Build history of the part. All positions in model axes, mm. Face numbers are marked on the shaded views. A direction names the side the tool comes from. Give positions to 0.01 mm unless a question says otherwise; leave off trailing zeros. Order: outer loops, then holes, each group sorted by start corner. A loop starts at its lowest first (then second) coordinate and runs counter-clockwise, first axis right, second up. Notation, with made-up numbers: (87.5, 14.25) - (129.5, 14.25) arc R21 cw to (129.5, 41.25) - close; hole circle Ø6 at (-13, 36.25). An arc over 180 degrees is marked (long way). Write each question's results on one line, items separated by ' | '. Start each with the question number.
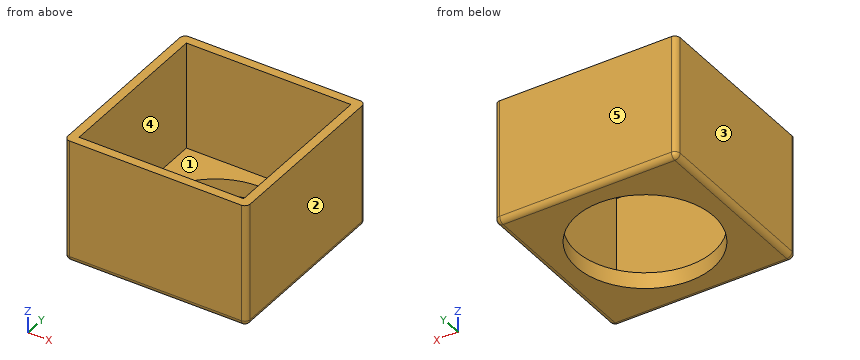
from build123d import *

# Parameters (mm, degrees)
F0_W     = 34
F0_H     = 34
F0_W_2   = 30.67
F0_H_2   = 30.67
F0_R     = 14.3
F0_R_2   = 12.8
F1_DEPTH = 3
F2_DEPTH = 20
F3_R     = 1


with BuildPart() as f1:
    # F0 (on Top) → F1 (new body)
    with BuildSketch(Plane.XY):
        Rectangle(F0_W, F0_H)
        Rectangle(F0_W_2, F0_H_2, mode=Mode.SUBTRACT)
        Rectangle(F0_W_2, F0_H_2)
        Circle(F0_R, mode=Mode.SUBTRACT)
        Circle(F0_R)
        Circle(F0_R_2, mode=Mode.SUBTRACT)
    extrude(amount=-F1_DEPTH)

    # F0 (on Top) → F2 (join)
    with BuildSketch(Plane.XY):
        Rectangle(F0_W, F0_H)
        Rectangle(F0_W_2, F0_H_2, mode=Mode.SUBTRACT)
    extrude(amount=F2_DEPTH)

    # F3
    f3_edges = [f1.edges().sort_by_distance(p)[0] for p in [
        (17, 0, -3),
        (0, 17, -3),
        (-17, 0, -3),
        (0, -17, -3),
        (17, -17, 8.5),
        (17, 17, 8.5),
        (-17, 17, 8.5),
        (-17, -17, 8.5),
    ]]
    fillet(f3_edges, radius=F3_R)


solid = f1.part
Item 1: Two-plate mould, pull along X, no slides. Class the marked faces 1, 2 and 3: +X half, -X half, draft (parallel to the pull), parting line (faces both ways), or undercut.
Item 2: Probe line 1 along X through (y, z) = (6, 5) (3 decimals); line 2 along Y through (x, z) = (0, -1.55). List the from-to ranges inside material, lowest first. Write a range as from..to.
Item 3: Cut at D-D, the plane x = 14. List the corners of the cut face in (y, z) (3 decimals), then the cut area to 3 significant figures.
Item 4: Which spindle directions (+Z, -Z, +X, -X, +Y, -Y) get a long thin tool onto all of the face, cutting with end or side? Do the marked faces 4 and 5. Say none if no direction does.
Item 5: Cut at A-A, the plane x = 0. List the corners of the cut face in (y, z) (3 decimals), then the cut area to 3 significant figures.
Item 6: Flat gauge pin, fed straight in: pin 1 Ø3 at (x, y) = (12, -10) entering from +Z. Where does the tip first touch, or does it go through?
Item 7: Cut at C-C, the plane z = 6.5. List the corners of the cut face in (x, y) (3 decimals), then the cut area to 3 significant figures.
Values found:
1) face 1: undercut | face 2: +X half | face 3: -X half
2) line 1: x = -17..-15.335, 15.335..17 | line 2: y = -17..-12.8, 12.8..17
3) outline: (-17, -2) arc R1 ccw to (-16, -3) - (16, -3) arc R1 ccw to (17, -2) - (17, 20) - (15.335, 20) - (15.335, 0) - (-15.335, 0) - (-15.335, 20) - (-17, 20) - close | area: 168 mm2
4) face 4: +Z | face 5: +Z, -Z, +X, -X, +Y
5) outline: (-17, -2) arc R1 ccw to (-16, -3) - (-12.8, -3) - (-12.8, 0) - (-15.335, 0) - (-15.335, 20) - (-17, 20) - close; (12.8, -3) - (16, -3) arc R1 ccw to (17, -2) - (17, 20) - (15.335, 20) - (15.335, 0) - (12.8, 0) - close | area: 91.4 mm2
6) pin 1: stops at z = 0
7) outline: (-17, -16) arc R1 ccw to (-16, -17) - (16, -17) arc R1 ccw to (17, -16) - (17, 16) arc R1 ccw to (16, 17) - (-16, 17) arc R1 ccw to (-17, 16) - close; hole (-15.335, -15.335) - (15.335, -15.335) - (15.335, 15.335) - (-15.335, 15.335) - close | area: 214 mm2
